Check sheet for the modelled part. Datum: model origin and axes. Units: mm. A direction names the side the tool comes from. Give positions to 0.01 mm unless a question says otherwise; leave off trailing zeros. Write each loop counter-clockwise with the first axis right and the second up, starting at its lowest first coordinate (ties: lowest second). Pieces come first, ordered by that corner, then holes. Notation, with made-up numbers: M 55,67.25 L 107,67.25 A22 cw 107,101.25 Z; hole C 68,88 d10. An arc over 180 degrees is marked long. Write item = value, one per line. Start each with the question number.
1) Mould release check, pull along X, two halves, no side actions. Record for faces 1 (the flat face through (-8.89, 0, 0)), 2 (the flat face through (1.714, 0, 0)), 3 (the flat face through (0, 0, 19.05)): released by +X, released by -X, zero draft, split by the parting line, or undercut.
2) Cross-section at C-C, the plane x = 0. Record the cut outline in (y, z), plus the area to 3 significant figures.
3) Access from +Z, -Z, +X, -X, +Y, -Y to the whole of each face (thin tool, end or side, straight path). Record for faces 4 (the flat face through (2, -1.397, 0)), 5 (the cylindrical face through (0.038, 0.02, 6.477)).
4) Cross-section at A-A, the plane z = 2.5. Record the cut outline in (x, y), plus the area to 3 significant figures.
5) Cross-section at B-B, the plane y = -0.6. Record the cut outline in (x, z), plus the area to 3 significant figures.
6) Scan lines: line 1 along X through (y, z) = (0.95, -1); line 2 along Z through (x, y) = (0, 0.8); line 3 along Z through (x, y) = (0.75, -0.3). Record each from-to range of solid material in increasing order. Write a range as [from, to].
```python
from build123d import *

# Parameters (mm, degrees)
SKETCH1_W           = 17.78
SKETCH1_H           = 2.794
BOSS_EXTRUDE1_DEPTH = 19.05
CUT_EXTRUDE1_DEPTH  = 22.207098717


with BuildPart() as part:
    # Sketch1 → Boss-Extrude1 (new, symmetric)
    with BuildSketch(Plane.XY):
        Rectangle(SKETCH1_W, SKETCH1_H)
    extrude(amount=BOSS_EXTRUDE1_DEPTH, both=True)

    # Sketch2 → Cut-Extrude1 (cut, through all)
    with BuildSketch(Plane(origin=(0, 1.397, 0), x_dir=(1, 0, 0), z_dir=(0, 1, 0))):
        with BuildLine():
            Line((-1.7145, -4.7625), (-1.7145, 4.7625))
            ThreePointArc((-1.7145, 4.7625), (0, 6.477), (1.7145, 4.7625))
            Line((1.7145, 4.7625), (1.7145, -4.7625))
            ThreePointArc((1.7145, -4.7625), (0, -6.477), (-1.7145, -4.7625))
        make_face()
    extrude(amount=-CUT_EXTRUDE1_DEPTH, mode=Mode.SUBTRACT)


solid = part.part
```
Reply:
q1.face_1 = released by -X
q1.face_2 = undercut
q1.face_3 = zero draft
q2.outline = M -1.4,-19.05 L 1.4,-19.05 L 1.4,-6.48 L -1.4,-6.48 Z; M -1.4,6.48 L 1.4,6.48 L 1.4,19.05 L -1.4,19.05 Z
q2.area = 70.3 mm2
q3.face_4 = +Z, -Z, +X, -X, -Y
q3.face_5 = +Y, -Y
q4.outline = M -8.89,-1.4 L -1.71,-1.4 L -1.71,1.4 L -8.89,1.4 Z; M 1.71,-1.4 L 8.89,-1.4 L 8.89,1.4 L 1.71,1.4 Z
q4.area = 40.1 mm2
q5.outline = M -8.89,-19.05 L 8.89,-19.05 L 8.89,19.05 L -8.89,19.05 Z; hole M -1.71,-4.76 A1.71 ccw 1.71,-4.76 L 1.71,4.76 A1.71 ccw -1.71,4.76 Z
q5.area = 636 mm2
q6.line_1 = [-8.89, -1.71], [1.71, 8.89]
q6.line_2 = [-19.05, -6.48], [6.48, 19.05]
q6.line_3 = [-19.05, -6.3], [6.3, 19.05]
